Check sheet for the modelled part. Datum: model origin and axes. Units: mm. Face numbers are marked on the shaded views. A direction names the side the tool comes from. Give positions to 0.01 mm unless a question says otherwise; leave off trailing zeros. Write each loop counter-clockwise with the first axis right and the second up, starting at its lowest first coordinate (ties: lowest second). Pieces come first, ordered by that corner, then holes. Notation, with made-up numbers: (60, -31) - (106, -31) arc R19 ccw to (106, -4) - close; hole circle Ø3 at (20, 59.5). An arc over 180 degrees is marked (long way). Return JSON: item names as keys, results as strings. Group by question number.
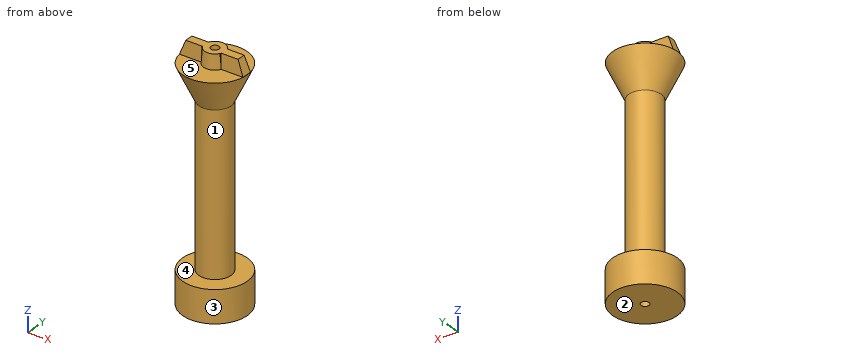
```python
from build123d import *

# Parameters (mm, degrees)
F3_DEPTH  = 4.5
F6_DEPTH  = 7.82
F9_DEPTH  = 7.71
F12_DEPTH = 25


with BuildPart() as f1:
    # F0 (on Front) → F1 (revolve)
    with BuildSketch(Plane.XZ):
        Polygon((-10, 0), (-1.25, 0), (-1.25, 74.5), (-3.15, 74.5), (-3.5, 70), (-10, 70), (-5, 59.2774653975), (-5, 10), (-10, 10), align=None)
    revolve(axis=Axis((0, 0, 54.2438514531), (0, 0, 1)))

    # F2 (on face) → F3 (join)
    with BuildSketch(Plane.XY.offset(70)):
        with BuildLine():
            Line((-3.1128764833, 1.6), (-9.8711701434, 1.6))
            ThreePointArc((-9.8711701434, 1.6), (-10, 0), (-9.8711701434, -1.6))
            Line((-9.8711701434, -1.6), (-3.1128764833, -1.6))
            Line((-3.1128764833, -1.6), (-2.7133927102, -1.6))
            ThreePointArc((-2.7133927102, -1.6), (-3.15, 0), (-2.7133927102, 1.6))
            Line((-2.7133927102, 1.6), (-3.1128764833, 1.6))
        make_face()
        with BuildLine():
            Line((9.8711701434, 1.6), (3.1128764833, 1.6))
            Line((3.1128764833, 1.6), (2.7133927102, 1.6))
            ThreePointArc((2.7133927102, 1.6), (3.15, 0), (2.7133927102, -1.6))
            Line((2.7133927102, -1.6), (3.1128764833, -1.6))
            Line((3.1128764833, -1.6), (9.8711701434, -1.6))
            ThreePointArc((9.8711701434, -1.6), (10, 0), (9.8711701434, 1.6))
        make_face()
    extrude(amount=F3_DEPTH)

    # F5 (on offset) → F6 (cut)
    with BuildSketch(Plane.YZ.offset(10.7)):
        Polygon((-1.6, 70), (-1.3, 74.5), (-1.6, 74.5), align=None)
        Polygon((1.6, 74.5), (1.3, 74.5), (1.6, 70), align=None)
    extrude(amount=-F6_DEPTH, mode=Mode.SUBTRACT)

    # F8 (on offset) → F9 (cut)
    with BuildSketch(Plane.YZ.offset(-10.7)):
        Polygon((1.6, 70), (1.6, 74.5), (1.3, 74.5), align=None)
        Polygon((-1.3, 74.5), (-1.6, 74.5), (-1.6, 70), align=None)
    extrude(amount=F9_DEPTH, mode=Mode.SUBTRACT)

    # F11 (on offset) → F12 (cut)
    with BuildSketch(Plane.XZ.offset(10)):
        Polygon((-10.2594941854, 70), (-9.8711701434, 70), (-7.9456651583, 74.9055147171), (-10.5508649722, 74.9055147171), align=None)
        Polygon((7.9456651583, 74.9055147171), (9.8711701434, 70), (10.2594941854, 70), (10.5508649722, 74.9055147171), align=None)
    extrude(amount=-F12_DEPTH, mode=Mode.SUBTRACT)


solid = f1.part
```
Item 1: Mould release check, pull along Z, two halves, no side actions. Record for the marked faces 3, 4 and 5: +Z half, -Z half, draft (parallel to the pull), parting line (faces both ways), or undercut.
Item 2: Access from +Z, -Z, +X, -X, +Y, -Y to the whole of each face (thin tool, end or side, straight path). Record for the marked faces 1 and 2.
Item 3: Depth check by flat-ended pin: pin 1 (4 mm diameter, centred on x = -1, y = -7.5, fed in from +Z); pin 2 (2 mm diameter, centred on x = -3, z = 14.5, fed in from +Y); pin 3 (5 mm diameter, centred on x = 3.5, z = 33, fed in from -Y). Enter the tip coordinate at first touch or a pass-through.
Item 4: Section check C-C on z = 22. Record the cut outline in (x, y).
Item 5: Section check A-A on y = 0. Record the cut outline in (x, z).
Item 6: Section check B-B on x = 0. Record the cut outline in (y, z).
Item 7: Material ranges on line 1 along Y through (x, z) = (0, 40.5); line 2 along Z through (x, y) = (1, 8.25), recorded low to high. Write a range as from..to.
Reply:
{
 "1": {"face 3": "draft", "face 4": "undercut", "face 5": "+Z half"},
 "2": {"face 1": "none", "face 2": "-Z, +X, -X, +Y, -Y"},
 "3": {"pin 1": "z = 70", "pin 2": "y = 4.58", "pin 3": "y = -4.9"},
 "4": {"outline": "circle Ø10 at (0, 0); hole circle Ø2.5 at (0, 0)"},
 "5": {"outline": "(-10, 0) - (-1.25, 0) - (-1.25, 74.5) - (-8.1, 74.5) - (-9.87, 70) - (-10, 70) - (-5, 59.28) - (-5, 10) - (-10, 10) - close; (1.25, 0) - (10, 0) - (10, 10) - (5, 10) - (5, 59.28) - (10, 70) - (9.87, 70) - (8.1, 74.5) - (1.25, 74.5) - close"},
 "6": {"outline": "(-10, 0) - (-1.25, 0) - (-1.25, 74.5) - (-3.15, 74.5) - (-3.5, 70) - (-10, 70) - (-5, 59.28) - (-5, 10) - (-10, 10) - close; (1.25, 0) - (10, 0) - (10, 10) - (5, 10) - (5, 59.28) - (10, 70) - (3.5, 70) - (3.15, 74.5) - (1.25, 74.5) - close"},
 "7": {"line 1": "-5..-1.25, 1.25..5", "line 2": "0..10, 66.38..70"}
}
